```python
from build123d import *

# Parameters (mm, degrees)
BOSS_EXTRUDE1_DEPTH = 20
CIRPATTERN1_COUNT   = 5
CIRPATTERN1_ANGLE   = 130


with BuildPart() as part:
    # Sketch1 → Boss-Extrude1 (new body)
    with BuildSketch(Plane.XY):
        with BuildLine():
            Line((-150, 0), (0, 0))
            ThreePointArc((0, 0), (-75, -75), (-150, 0))
        make_face()
    extrude(amount=BOSS_EXTRUDE1_DEPTH)

    # Sketch4 → Ø4.0mm Dowel Hole2 (revolve, cut)
    with BuildSketch(Plane(origin=(-7.026915972, -31.696369631, 10), x_dir=(0.4226182617407001, 0.9063077870366498, 0), z_dir=(0, 0, 1))):
        Polygon((0, 0), (0, 17.201721238), (2, 16), (2, 0.025), (2.025, 0), align=None)
    f_4_0mm_dowel_hole2 = revolve(axis=Axis((-1.271861525, -34.379995593, 10), (-0.9063077870366497, 0.42261826174070016, 0)), mode=Mode.SUBTRACT)

    # CirPattern1: Ø4.0mm Dowel Hole2 ×5 about axis
    cirpattern1_axis = Axis((-75, 0, 0), (0, 0, -1))
    for i in range(1, CIRPATTERN1_COUNT):
        add(f_4_0mm_dowel_hole2.rotate(cirpattern1_axis, i * CIRPATTERN1_ANGLE / (CIRPATTERN1_COUNT - 1)), mode=Mode.SUBTRACT)


solid = part.part
```
Check sheet for the modelled part. Datum: model origin and axes. Units: mm. A direction names the side the tool comes from. Round coordinates to 2 decimals unless told otherwise and drop trailing zeros. Order: outer loops, then holes, each group sorted by start corner. A loop starts at its lowest first (then second) coordinate and runs counter-clockwise, first axis right, second up.
1) Mould release check, pull along Y, two halves, no side actions. Record for faces 4 (the flat face through (-74, -29, 20)), 5 (the cylindrical face through (-15.03, -30.17, 9.91)), 6 (the cylindrical face through (-135.01, -30.09, 9.4)), 7 (the flat face through (-76, 0, 10)): +Y half, -Y half, draft (parallel to the pull), parting line (faces both ways), or undercut.
2) Tool access check on faces 1 (the cylindrical face through (-73.35, -74.98, 7.64)), 2 (the conical face through (-43.553, -48.745, 9.896)), 3 (the cylindrical face through (-77, -67, 10)). Record the directions out of +Z, -Z, +X, -X, +Y, -Y that give a thin tool (end or side, any length) a straight path to the whole face; none if there is none.
3) Scan lines: line 1 (Z direction, x = -75, y = -63); line 2 (X direction, y = -67.5, z = 9.75); line 3 (X direction, y = -65.5, z = 10). Record each from-to range of solid material in increasing order.
4) Section check A-A (z = 6.25). Record the boundary of the cut face in (x, y), and give its area (3 significant figures).
5) Go/stop test with flat-tipped pins: pin 1 Ø3 at (y, z) = (-31.5, 3.5) entering from +X; pin 2 Ø1.5 at (y, z) = (-44.5, 12.5) entering from +X; pin 3 Ø6 at (y, z) = (-9, 7) entering from +X. Record where each tip stops, or that it passes through.
6) Section check B-B (x = -54). Record the boundary of the cut face in (y, z).
7) Section check C-C (y = -16). Record the boundary of the cut face in (x, z), and give its area (3 significant figures).
Result:
1. face 4: draft
1. face 5: undercut
1. face 6: undercut
1. face 7: +Y half
2. face 1: +Z, -Z, -Y
2. face 2: none
2. face 3: -Y
3. line 1: z = 0 to 8, 12 to 20
3. line 2: x = -107.69 to -76.98, -73.02 to -42.31
3. line 3: x = -111.53 to -77, -73 to -38.47
4. outline: (-150, 0) arc R75 ccw to (0, 0) - close
4. area: 8,840 mm2
5. pin 1: stops at x = -6.26
5. pin 2: stops at x = -14.08
5. pin 3: stops at x = -0.24
6. outline: (-72, 0) - (0, 0) - (0, 20) - (-72, 20) - close
7. outline: (-148.27, 0) - (-1.73, 0) - (-1.73, 20) - (-148.27, 20) - close
7. area: 2,930 mm2
